Build history of the part. All positions in model axes, mm. Coordinates: 2 decimals unless noted, no trailing zeros. Loops run counter-clockwise (first coordinate to the right, second up) from the corner with the lowest first, then second, coordinate; pieces in that order, holes last.
(1) Slice it at A-A (x = -49). Give the cut face in (y, z).
(2) Wall check: L1, parallel to X at y = 160, z = 0 (3 decimals); L2, parallel to Z at x = -21, y = 90; L3, parallel to X at y = -215, z = 5. Give the ranges that are in metal, low to high.
(3) Flat gauge pins, fed straight in: P1, Ø1, axis at x = 13.5, y = -209.5, coming from the -Z side; P2, Ø2, axis at y = 48.5, z = -13, coming from the +X side; P3, Ø4, axis at x = 4, y = -46.5, coming from the -Z side. Where does each tip first touch, or does it go through?
(4) Slice it at C-C (y = 62.5). Give the cut face in (x, z) (3 decimals).
(5) Slice it at B-B (z = -14.5). Give the cut face in (x, y).
from build123d import *

# Parameters (mm, degrees)
SKETCH1_R           = 65.405
SKETCH1_R_2         = 63.5
BOSS_EXTRUDE1_DEPTH = 342.9
SKETCH4_W           = 3.175
SKETCH4_H           = 203.2
CUT_EXTRUDE2_DEPTH  = 66.405
CIRPATTERN4_COUNT   = 2
CIRPATTERN4_ANGLE   = 90


with BuildPart() as part:
    # Sketch1 → Boss-Extrude1 (new body, symmetric)
    with BuildSketch(Plane(origin=(0, 0, 0), x_dir=(1, 0, 0), z_dir=(0, 1, 0))):
        Circle(SKETCH1_R)
        Circle(SKETCH1_R_2, mode=Mode.SUBTRACT)
    extrude(amount=BOSS_EXTRUDE1_DEPTH, both=True)

    # Sketch4 → Cut-Extrude2 (cut, symmetric)
    with BuildSketch(Plane(origin=(0, 0, 0), x_dir=(0, 0, -1), z_dir=(1, 0, 0))):
        with Locations((0, -190.5)):
            Rectangle(SKETCH4_W, SKETCH4_H)
    cut_extrude2 = extrude(amount=CUT_EXTRUDE2_DEPTH, both=True, mode=Mode.SUBTRACT)

    # CirPattern4: Cut-Extrude2 ×2 about axis
    cirpattern4_axis = Axis((0, 342.9, 0), (0, -1, 0))
    for i in range(1, CIRPATTERN4_COUNT):
        add(cut_extrude2.rotate(cirpattern4_axis, i * CIRPATTERN4_ANGLE / (CIRPATTERN4_COUNT - 1)), mode=Mode.SUBTRACT)


solid = part.part
Response values:
1. outline: (-342.9, -43.32) - (342.9, -43.32) - (342.9, -40.39) - (-342.9, -40.39) - close; (-342.9, 40.39) - (342.9, 40.39) - (342.9, 43.32) - (-342.9, 43.32) - close
2. L1: x = -65.405 to -63.5, 63.5 to 65.405
2. L2: z = -61.94 to -59.93, 59.93 to 61.94
2. L3: x = -65.21 to -63.3, 63.3 to 65.21
3. P1: stops at z = -64.1
3. P2: stops at x = 64.29
3. P3: stops at z = -65.37
4. outline: circle Ø130.81 at (0, 0); hole circle Ø127 at (0, 0)
5. outline: (-63.78, -342.9) - (-61.82, -342.9) - (-61.82, 342.9) - (-63.78, 342.9) - close; (61.82, -342.9) - (63.78, -342.9) - (63.78, 342.9) - (61.82, 342.9) - close
